Check sheet for the drawn part. Datum: minimum x, y, z corner. Units: mm. A direction names the side the tool comes from. Round coordinates to 2 decimals unless told otherwise and drop trailing zeros. Write each loop counter-clockwise with the first axis right and the second up, starting at its lowest first coordinate (ties: lowest second). Pieces come first, ordered by that corner, then holes.
Item 1: Cross-section at A-A on z = 55. Enter the section's corners in (x, y), plus the area to 3 significant figures.
Item 2: Go/stop test with flat-tipped pins: pin 1 Ø15 at (x, y) = (40.5, 51) entering from +Z; pin 2 Ø2 at (x, z) = (54, 34) entering from -Y; pin 3 Ø7.5 at (y, z) = (8.5, 37.5) entering from -X; pin 4 Ø5 at (y, z) = (43.5, 55.5) entering from -X. Record where each tip stops, or that it passes through.
Item 3: Cross-section at B-B on y = 51.5. Enter the section's corners in (x, z).
Item 4: Cross-section at C-C on x = 57.5. Enter the section's corners in (y, z), plus the area to 3 significant figures.
Item 5: Cross-section at D-D on x = 20.5. Enter the section's corners in (y, z).
Item 6: Material ranges on line 1 (Z direction, x = 61, y = 36.5); line 2 (Y direction, x = 24, z = 45.5); line 3 (X direction, y = 11.5, z = 43), recorded low to high.
Item 7: Tool access check on the marked faces 1, 2, 3 and 4. Record the directions out of +Z, -Z, +X, -X, +Y, -Y that give a thin tool (end or side, any length) a straight path to the whole face; none if there is none.
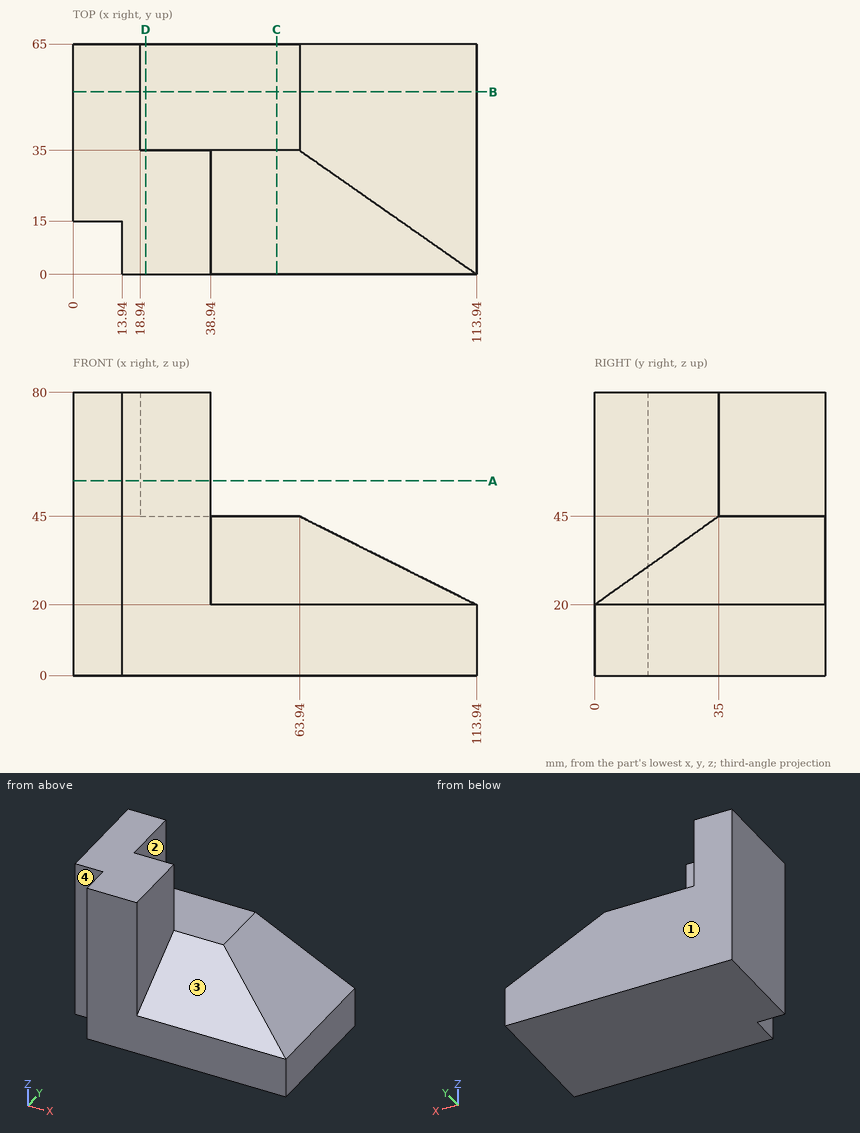
Response values:
1. outline: (0, 15) - (13.94, 15) - (13.94, 0) - (38.94, 0) - (38.94, 35) - (18.94, 35) - (18.94, 65) - (0, 65) - close
1. area: 1,720 mm2
2. pin 1: stops at z = 45
2. pin 2: stops at y = 18.2
2. pin 3: stops at x = 13.94
2. pin 4: stops at x = 0
3. outline: (0, 0) - (113.94, 0) - (113.94, 20) - (63.94, 45) - (18.94, 45) - (18.94, 80) - (0, 80) - close
4. outline: (0, 0) - (65, 0) - (65, 45) - (35, 45) - (0, 20) - close
4. area: 2,490 mm2
5. outline: (0, 0) - (65, 0) - (65, 45) - (35, 45) - (35, 80) - (0, 80) - close
6. line 1: z = 0 to 45
6. line 2: y = 0 to 35
6. line 3: x = 13.94 to 38.94
7. face 1: +Z, -Z, +X, -X, +Y
7. face 2: +Z, +X, +Y
7. face 3: +Z, +X, -Y
7. face 4: +Z, -Z, -X, -Y
